Design review of the part built by this model. Coordinates are the model's own, in mm. Face numbers are marked on the shaded views. A direction names the side the tool comes from. Give positions to 0.01 mm unless a question says otherwise; leave off trailing zeros. Write each loop counter-clockwise with the first axis right and the second up, starting at its lowest first coordinate (ties: lowest second). Pieces come first, ordered by that corner, then holes. Notation, with made-up numbers: (-6, 70) - (20, 70) arc R14 ccw to (20, 89) - close; hole circle Ø6 at (25.25, 16.5). An arc over 180 degrees is marked (long way). Use a Markdown table: item, result. Add a question column.
```python
from build123d import *

# Parameters (mm, degrees)
SKETCH2_W          = 2
SKETCH2_H          = 2
REVOLVE2_ANGLE     = 20
SKETCH3_W          = 2.2
SKETCH3_H          = 6.8
CUT_REVOLVE1_ANGLE = 25
SKETCH4_W          = 4.7
SKETCH4_H          = 2.5
CUT_REVOLVE2_ANGLE = 45


with BuildPart() as part:
    # Sketch1 → Revolve1 (revolve)
    with BuildSketch(Plane.XY, mode=Mode.PRIVATE) as revolve1_sk:
        Polygon((12, 15), (12, -5), (14.5, -5), (14.5, -15), (17.5, -15), (17.5, -5), (15.190598923, -1), (17.5, 3), (17.5, 5), (14, 5), (14, 15), align=None)
    revolve(revolve1_sk.sketch.rotate(Axis((0, 40.467735012, 0), (0, -1, 0)), 90), axis=Axis((0, 40.467735012, 0), (0, -1, 0)))

    # Sketch2 → Revolve2 (revolve, symmetric)
    with BuildSketch(Plane.XY) as revolve2_sk:
        with Locations((15, 11)):
            Rectangle(SKETCH2_W, SKETCH2_H)
        with Locations((-15, 11)):
            Rectangle(SKETCH2_W, SKETCH2_H)
    revolve(axis=Axis((0, 45.306661743, 0), (0, -1, 0)), revolution_arc=REVOLVE2_ANGLE / 2)
    revolve(revolve2_sk.sketch, axis=Axis((0, 45.306661743, 0), (0, 1, 0)), revolution_arc=REVOLVE2_ANGLE / 2)

    # Sketch3 → Cut-Revolve1 (revolve, symmetric, cut)
    with BuildSketch(Plane.XY) as cut_revolve1_sk:
        with Locations((-15.6, -11.6)):
            Rectangle(SKETCH3_W, SKETCH3_H)
        with Locations((15.6, -11.6)):
            Rectangle(SKETCH3_W, SKETCH3_H)
    revolve(axis=Axis((0, -11.020729768, 0), (0, -1, 0)), revolution_arc=CUT_REVOLVE1_ANGLE / 2, mode=Mode.SUBTRACT)
    revolve(cut_revolve1_sk.sketch, axis=Axis((0, -11.020729768, 0), (0, 1, 0)), revolution_arc=CUT_REVOLVE1_ANGLE / 2, mode=Mode.SUBTRACT)

    # Sketch4 → Cut-Revolve2 (revolve, cut)
    with BuildSketch(Plane.XY):
        with Locations((-14.35, -9.45)):
            Rectangle(SKETCH4_W, SKETCH4_H)
        with Locations((14.35, -9.45)):
            Rectangle(SKETCH4_W, SKETCH4_H)
    revolve(axis=Axis((0, -42.004114959, 0), (0, 1, 0)), revolution_arc=CUT_REVOLVE2_ANGLE, mode=Mode.SUBTRACT)


solid = part.part
```
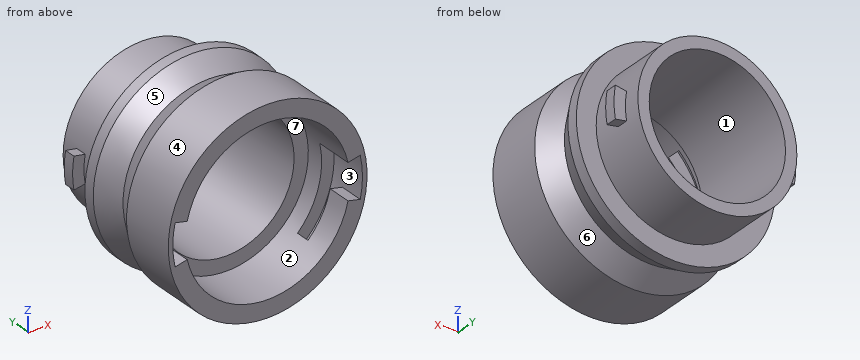
(1) Add section B-B (y = 4). State the section outline as (x, z) points.
(2) Add section C-C (x = 0). State the section outline as (y, z) points, and give its area (3 significant figures).
(3) For line 1 along X through (y, z) = (4.75, 0); line 2 along X through (y, z) = (-10, 11.5); line 3 along X through (y, z) = (9.5, 0), list the stretches that pass through material, from the lowest coordinate up.
(4) Tool access review of the marked faces 1, 2 and 3: name each direction out of +Z, -Z, +X, -X, +Y, -Y from which nothing blocks a thin tool from reaching the whole face with its end or side.
(5) Insertion check: pin 1 (0.7 mm diameter, centred on x = -15.5, z = 0.5, fed in from +Y); pin 2 (1.8 mm diameter, centred on x = 12.5, z = -9, fed in from +Y); pin 3 (4 mm diameter, centred on y = 10.5, z = 9, fed in from -X). Each pin has a flat end and moves straight along its axis. Give the tip position at first contact, or say it passes through.
(6) Mouldability with a two-part tool opening along Y and no side actions: class the marked faces 4, 5, 6 and 7 as +Y half, -Y half, draft (parallel to the pull), parting line (faces both ways), or undercut.
Answers follow:
| question | item | result |
|---|---|---|
| 1 | outline | circle Ø35 at (0, 0); hole circle Ø24 at (0, 0) |
| 2 | outline | (-15, -17.5) - (-5, -17.5) - (-1, -15.19) - (3, -17.5) - (5, -17.5) - (5, -14) - (15, -14) - (15, -12) - (-5, -12) - (-5, -14.5) - (-15, -14.5) - close; (-15, 14.5) - (-5, 14.5) - (-5, 12) - (15, 12) - (15, 14) - (5, 14) - (5, 17.5) - (3, 17.5) - (-1, 15.19) - (-5, 17.5) - (-15, 17.5) - close |
| 2 | area | 192 mm^2 |
| 3 | line 1 | -17.5 to -12, 12 to 17.5 |
| 3 | line 2 | -13.19 to -12.11, -11.5 to -8.83, 8.83 to 13.19 |
| 3 | line 3 | -14 to -12, 12 to 14 |
| 4 | face 1 | +Y, -Y |
| 4 | face 2 | -Y |
| 4 | face 3 | none |
| 5 | pin 1 | y = 12 |
| 5 | pin 2 | y = 5 |
| 5 | pin 3 | x = -12.12 |
| 6 | face 4 | draft |
| 6 | face 5 | undercut |
| 6 | face 6 | undercut |
| 6 | face 7 | -Y half |
